Job drawing, mm, ordinate dimensions from the low corner. One solid piece. Round coordinates to 2 decimals unless told otherwise and drop trailing zeros. Loops run counter-clockwise (first coordinate to the right, second up) from the corner with the lowest first, then second, coordinate; pieces in that order, holes last. Notation, with made-up numbers: M 6.25,-29 L 49.25,-29 A21 ccw 49.25,-17 Z; hole C -3.75,14 d10. An arc over 180 degrees is marked long. One line per item, written item: value.
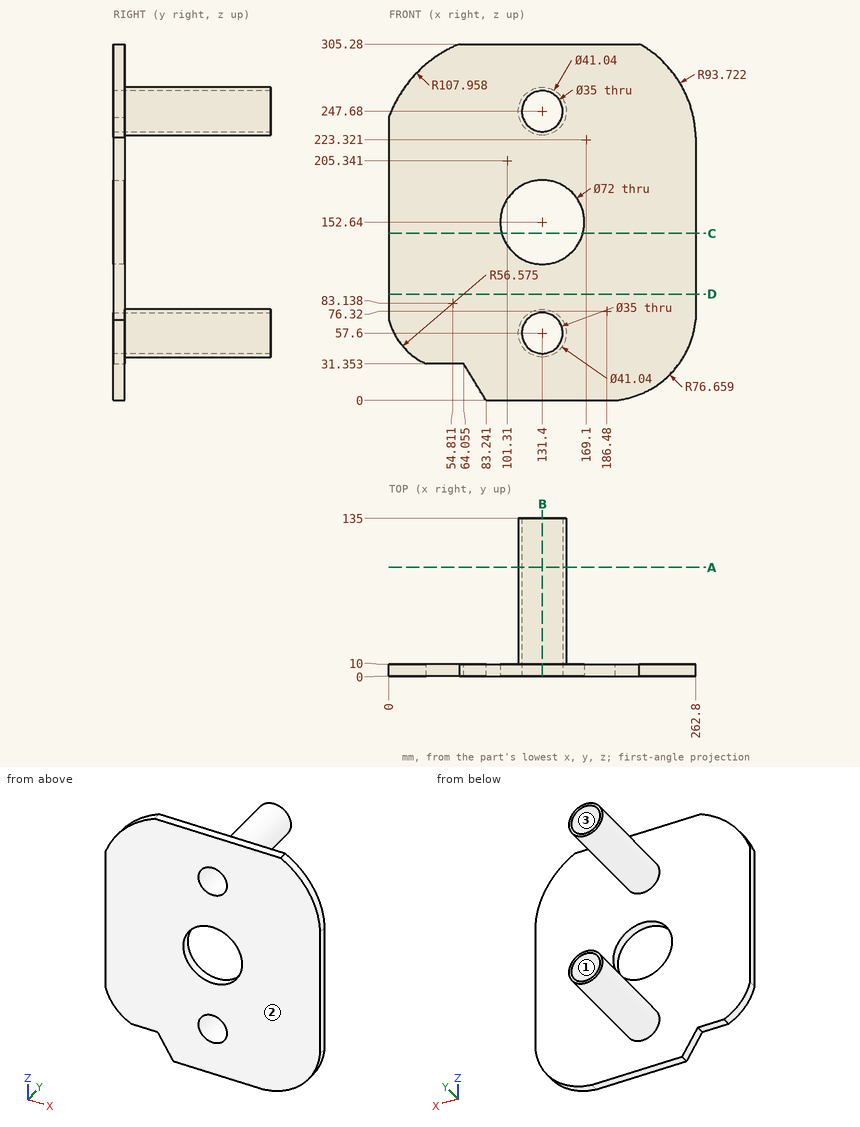
Item 1: Wall check: line 1 along Z through (x, y) = (131, 57) (1 decimal); line 2 along Z through (x, y) = (131, 6) (1 decimal); line 3 along X through (y, z) = (7, 152) (1 decimal). Give the ranges that are in metal, low to high.
Check values:
line 1: z = 37.1 to 40.1, 75.1 to 78.1, 227.2 to 230.2, 265.2 to 268.2
line 2: z = 0 to 40.1, 75.1 to 116.6, 188.6 to 230.2, 265.2 to 305.3
line 3: x = 0 to 95.4, 167.4 to 262.8
Item 2: Slice it at C-C, the plane z = 143. Give the cut face in (x, y) (1 decimal).
Check values:
outline: M 0,0 L 96.7,0 L 96.7,10 L 0,10 Z; M 166.1,0 L 262.8,0 L 262.8,10 L 166.1,10 Z
Item 3: Slice it at A-A, the plane y = 93. Give the cut face in (x, z).
Check values:
outline: C 131.4,57.6 d41.04; C 131.4,247.68 d41.04; hole C 131.4,57.6 d35; hole C 131.4,247.68 d35
Item 4: Slice it at D-D, the plane z = 91. Give the cut face in (x, y).
Check values:
outline: M 0,0 L 262.8,0 L 262.8,10 L 0,10 Z
Item 5: Drop flat-ended pins along their axis: P1, Ø3, axis at x = 168.5, z = 102, coming from the +Y side; P2, Ø5, axis at x = 42, y = 4.5, coming from the -Z side; P3, Ø1.5, axis at x = 125.5, y = 69, coming from the -Z side. Give the stop position or say it passes through.
Check values:
P1: stops at y = 10
P2: stops at z = 31.35
P3: stops at z = 37.74
Item 6: Slice it at B-B, the plane x = 131.4. Give the cut face in (y, z).
Check values:
outline: M 0,0 L 10,0 L 10,37.08 L 135,37.08 L 135,40.1 L 0,40.1 Z; M 0,75.1 L 135,75.1 L 135,78.12 L 10,78.12 L 10,116.64 L 0,116.64 Z; M 0,188.64 L 10,188.64 L 10,227.16 L 135,227.16 L 135,230.18 L 0,230.18 Z; M 0,265.18 L 135,265.18 L 135,268.2 L 10,268.2 L 10,305.28 L 0,305.28 Z
Item 7: Pull direction Z, two halves, no side cores. Call the marked faces 1, 2 and 3: pulls with the +Z half, pulls with the -Z half, needs draft (parallel to the pull), parting line crosses it, or undercut.
Check values:
face 1: undercut
face 2: needs draft
face 3: undercut
